The figure shows three views and two pictorial views of one solid part (mm, origin at its lowest corner). Answer the questions. A direction names the side the tool comes from. Coordinates: 2 decimals unless noted, no trailing zeros. Order: outer loops, then holes, each group sorted by start corner. A loop starts at its lowest first (then second) coordinate and runs counter-clockwise, first axis right, second up. Notation, with made-up numbers: (-17, 50.5) -> (29, 50.5) arc R21 ccw to (29, 89.5) -> close; hole circle Ø6 at (17.25, -36.75). An arc over 180 degrees is marked (long way). Write item = value, one per line. Start each with the question number.
Q1. The part is cut by section D-D, the plane y = 120. Determine the outline of the cut face in (x, z).
Q2. Which of the six approach directions +Z, -Z, +X, -X, +Y, -Y give full straight-line access (tool end or side, diameter ignored) to the marked faces 3 and 4?
Q3. For a pull along X with two mould halves and no side action, classify the marked faces 1 and 2 as +X half, -X half, draft (parallel to the pull), parting line (faces both ways), or undercut.
Q4. The part is cut by section C-C, the plane x = 11.5. Determine the outline of the cut face in (y, z) (1 decimal).
Q5. Straight lines are drawn through the part: L1, parallel to Y at x = 19.05, z = 2; L2, parallel to Z at x = 16.5, y = 153.5; L3, parallel to Y at x = 31, z = 15.25 (1 decimal). For each, find the intervals that lie inside material, in ascending order. Write a range as from..to.
Q6. Flat-ended cylindrical pins translate along their axes: pin 1 (19 mm diameter, centred on x = 16, y = 101, fed in from +Z); pin 2 (7 mm diameter, centred on x = 19.05, y = 190.5, fed in from -Z); pin 3 (10 mm diameter, centred on x = 27, z = 18, fed in from +Y). Find the tip coordinate at first contact, or state that the pin passes through.
Q7. The part is cut by section B-B, the plane z = 18. Determine the outline of the cut face in (x, y) (1 decimal).
Q8. The part is cut by section A-A, the plane y = 190.5. Determine the outline of the cut face in (x, z), plus the area to 3 significant figures.
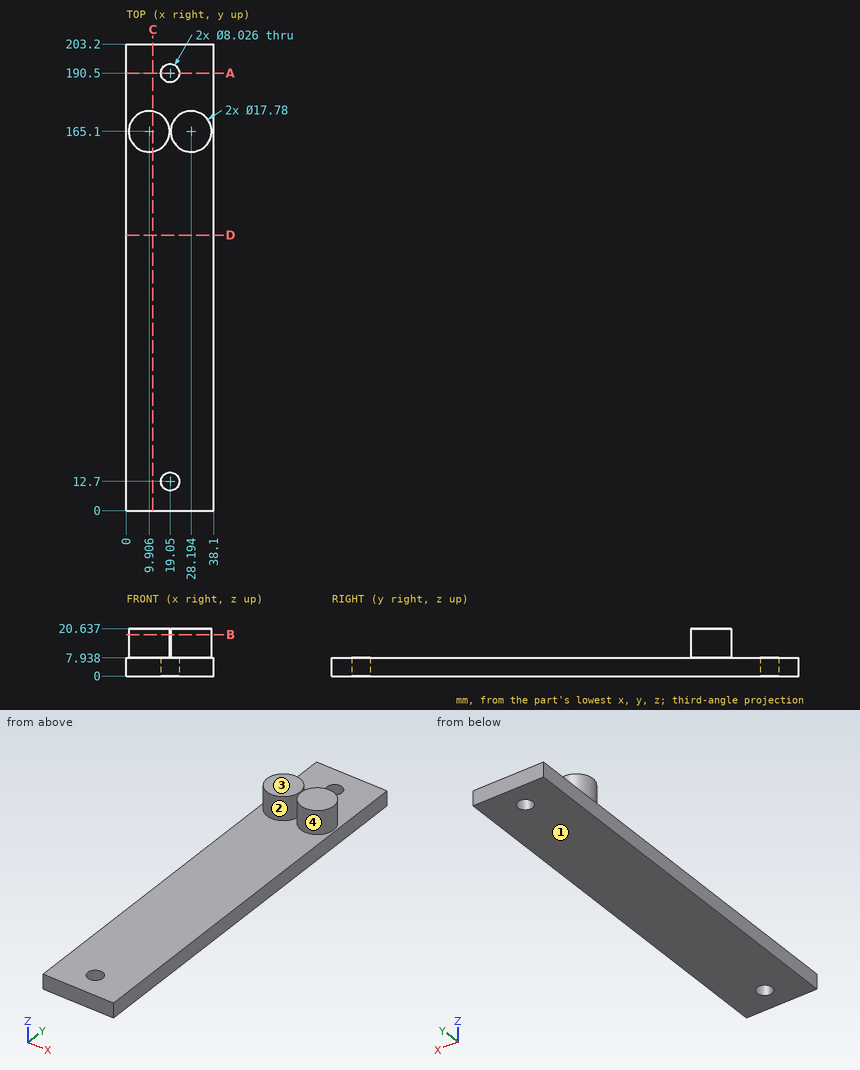
Model answer:
q1.outline = (0, 0) -> (38.1, 0) -> (38.1, 7.94) -> (0, 7.94) -> close
q2.face_3 = +Z, +X, -X, +Y, -Y
q2.face_4 = +Z
q3.face_1 = draft
q3.face_2 = undercut
q4.outline = (0, 0) -> (203.2, 0) -> (203.2, 7.9) -> (173.8, 7.9) -> (173.8, 20.6) -> (156.4, 20.6) -> (156.4, 7.9) -> (0, 7.9) -> close
q5.L1 = 0..8.69, 16.71..186.49, 194.51..203.2
q5.L2 = 0..7.94
q5.L3 = 156.7..173.5
q6.pin_1 = 7.94
q6.pin_2 = through
q6.pin_3 = 173.99
q7.outline = circle Ø17.8 at (9.9, 165.1); circle Ø17.8 at (28.2, 165.1)
q8.outline = (0, 0) -> (15.04, 0) -> (15.04, 7.94) -> (0, 7.94) -> close; (23.06, 0) -> (38.1, 0) -> (38.1, 7.94) -> (23.06, 7.94) -> close
q8.area = 239 mm2
